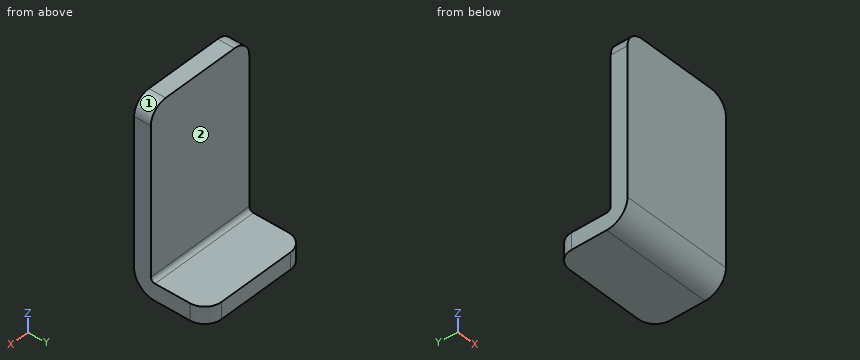
from build123d import *

# Parameters (mm, degrees)
BASE_FLANGE1_DEPTH = 20
FILLET1_R          = 3


# Sheet-metal steps are written as plain solids
with BuildPart() as part:
    # Sketch1 → Base-Flange1 (new body)
    with BuildSketch(Plane(origin=(0, 0, 0), x_dir=(0, 0, -1), z_dir=(1, 0, 0))):
        with BuildLine():
            Line((0, 0), (29.2634, 0))
            ThreePointArc((29.2634, 0), (29.784254855, 0.215745145), (30, 0.7366))
            Line((30, 0.7366), (30, 10))
            Line((30, 10), (33, 10))
            Line((33, 10), (33, 0.7366))
            ThreePointArc((33, 0.7366), (31.905575199, -1.905575199), (29.2634, -3))
            Line((29.2634, -3), (0, -3))
            Line((0, -3), (0, 0))
        make_face()
    extrude(amount=BASE_FLANGE1_DEPTH)

    # Fillet1
    fillet1_edges = [part.edges().sort_by_distance(p)[0] for p in [
        (20, -1.5, 0),
        (20, 10, -31.5),
        (0, -1.5, 0),
        (0, 10, -31.5),
    ]]
    fillet(fillet1_edges, radius=FILLET1_R)


solid = part.part
Read the model definition and answer for the solid it produces. Units are mm, in the model's axes. Face numbers are marked on the shaded views. A direction names the side the tool comes from. Give positions to 0.01 mm unless a question says otherwise; leave off trailing zeros. Write each loop counter-clockwise with the first axis right and the second up, starting at its lowest first coordinate (ties: lowest second). Pieces come first, ordered by that corner, then holes. Notation, with made-up numbers: (66.25, 60.5) - (112.25, 60.5) arc R8 ccw to (112.25, 64.5) - close; hole circle Ø11 at (31.25, -32.75). An arc over 180 degrees is marked (long way). Answer in a Markdown table with one row per item. Add a question column.
Item 1: A tool of negligible diameter and unlimited length cuts with its end or side. For the marked faces 1 and 2, from which of +Z, -Z, +X, -X, +Y, -Y can it reach the whole face along a straight path? Write none if from no direction.
Item 2: Section A-A, the plane x = 4.25 is taken. Write down the section's boundary in (y, z), and give its area (3 significant figures).
Item 3: Find the intervals of material crossed by L1, parallel to Z at x = 15, y = 1.75; L2, parallel to Y at x = 9.75, z = -7; L3, parallel to Z at x = 5.75, y = -2, in increasing order.
Item 4: Section B-B, the plane y = 5.5 is taken. Write down the section's boundary in (x, z), and give its area (3 significant figures).
Item 5: A flat-ended cylindrical pin translates along its axis: P1, Ø6, axis at y = 2.5, z = -8, coming from the -X side. Find the tip coordinate at first contact, or state that the pin passes through.
Item 6: Section D-D, the plane x = 18.5 is taken. Write down the section's boundary in (y, z), and give its area (3 significant figures).
Item 7: Section C-C, the plane z = -10.5 is taken. Write down the section's boundary in (x, y), and give its area (3 significant figures).
Recorded:
| question | item | result |
|---|---|---|
| 1 | face 1 | +Z, +X, +Y, -Y |
| 1 | face 2 | +Z, +X, -X, +Y |
| 2 | outline | (-3, -29.26) arc R3.74 ccw to (0.74, -33) - (10, -33) - (10, -30) - (0.74, -30) arc R0.74 cw to (0, -29.26) - (0, 0) - (-3, 0) - close |
| 2 | area | 126 mm2 |
| 3 | L1 | z = -33 to -30 |
| 3 | L2 | y = -3 to 0 |
| 3 | L3 | z = -31.81 to 0 |
| 4 | outline | (0, -33) - (20, -33) - (20, -30) - (0, -30) - close |
| 4 | area | 60.0 mm2 |
| 5 | P1 | stops at x = 0 |
| 6 | outline | (-3, -29.26) arc R3.74 ccw to (0.74, -33) - (9.6, -33) - (9.6, -30) - (0.74, -30) arc R0.74 cw to (0, -29.26) - (0, -0.4) - (-3, -0.4) - close |
| 6 | area | 124 mm2 |
| 7 | outline | (0, -3) - (20, -3) - (20, 0) - (0, 0) - close |
| 7 | area | 60.0 mm2 |
